Geometry check sheet. Reference: the model listing, model coordinates, mm. Round coordinates to 2 decimals unless told otherwise and drop trailing zeros. Write each loop counter-clockwise with the first axis right and the second up, starting at its lowest first coordinate (ties: lowest second). Pieces come first, ordered by that corner, then holes. Notation, with made-up numbers: (-6, 17) - (28, 17) arc R29 cw to (28, 44) - close; hole circle Ø7 at (75, 70.25). An arc over 180 degrees is marked (long way). Return JSON: item names as keys, results as strings. Group by question number.
from build123d import *

# Parameters (mm, degrees)
F0_W     = 60
F0_H     = 92.5
F0_R     = 2.5
F1_DEPTH = 2


with BuildPart() as f1:
    # F0 (on Top) → F1 (new body)
    with BuildSketch(Plane.XY):
        with Locations((0, -26.25)):
            Rectangle(F0_W, F0_H)
        with Locations((0, -52.5)):
            Circle(F0_R, mode=Mode.SUBTRACT)
        with Locations((0, -45)):
            Circle(F0_R, mode=Mode.SUBTRACT)
        with Locations((0, -37.5)):
            Circle(F0_R, mode=Mode.SUBTRACT)
        with Locations((0, -30)):
            Circle(F0_R, mode=Mode.SUBTRACT)
        with Locations((0, -22.5)):
            Circle(F0_R, mode=Mode.SUBTRACT)
        with Locations((0, -15)):
            Circle(F0_R, mode=Mode.SUBTRACT)
        with Locations((0, -7.5)):
            Circle(F0_R, mode=Mode.SUBTRACT)
        Circle(F0_R, mode=Mode.SUBTRACT)
    extrude(amount=F1_DEPTH)


solid = f1.part
1. Section check B-B (z = 0.3). State how many separate pieces and enclosed holes the cut face has, and give its area (3 significant figures).
2. Section check A-A (y = -52.5). Enter the section's corners in (x, z).
3. Material ranges on line 1 along X through (y, z) = (-29, 1.35); line 2 along X through (y, z) = (0.5, 1.8), recorded low to high.
4. Mould release check, pull along Y, two halves, no side actions. Record for faces 1 (the face through (0, -26, 0)), 2 (the face through (-0.54, -17.44, 0.99)), 3 (the face through (0, -72.5, 1)): pulls with the +Y half, pulls with the -Y half, needs draft (parallel to the pull), parting line crosses it, or undercut.
Result sheet:
{
 "1": {"separate pieces": "1", "enclosed holes": "8", "area": "5,390 mm²"},
 "2": {"outline": "(-30, 0) - (-2.5, 0) - (-2.5, 2) - (-30, 2) - close; (2.5, 0) - (30, 0) - (30, 2) - (2.5, 2) - close"},
 "3": {"line 1": "x = -30 to -2.29, 2.29 to 30", "line 2": "x = -30 to -2.45, 2.45 to 30"},
 "4": {"face 1": "needs draft", "face 2": "undercut", "face 3": "pulls with the -Y half"}
}
